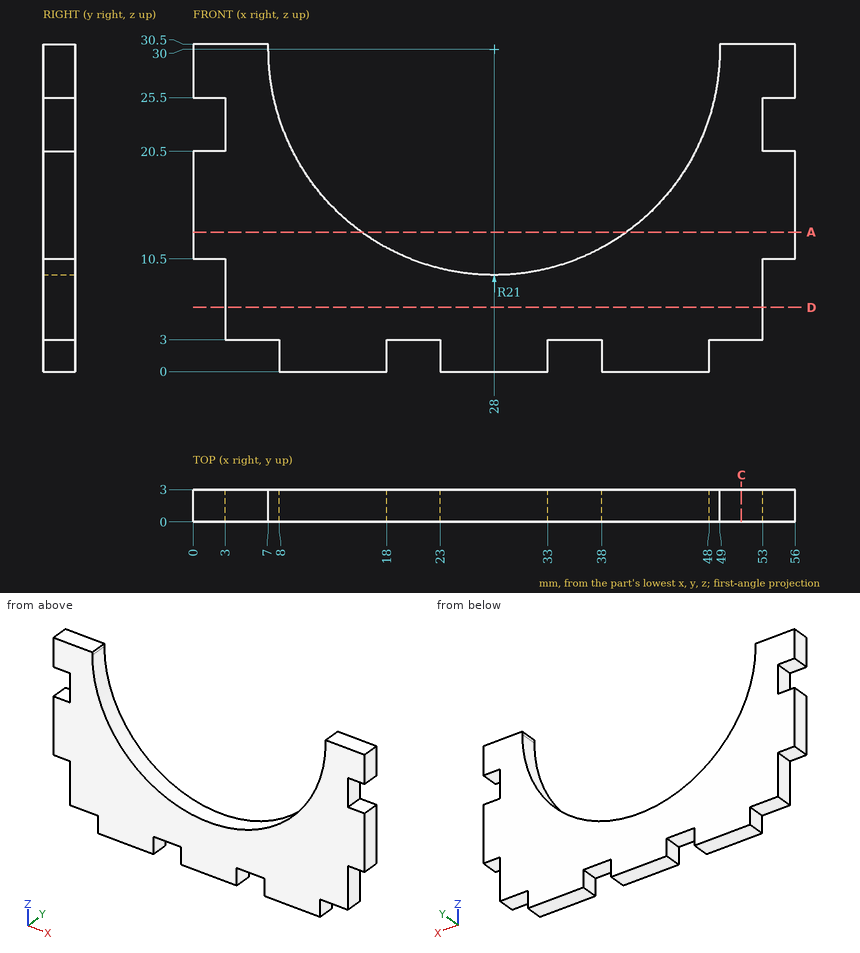
Print and shaded views of the part. All mm, measured from the part's lowest x, y and z. Round coordinates to 2 decimals unless told otherwise and drop trailing zeros. Write each loop counter-clockwise with the first axis right and the second up, starting at its lowest first coordinate (ties: lowest second). Pieces come first, ordered by that corner, then holes. Notation, with made-up numbers: (-1, 10) - (4, 10) arc R21 cw to (4, 27) - close; hole circle Ø7 at (30.25, -37.5). An arc over 180 degrees is marked (long way). Write each question's results on one line, items separated by ' | '. Start each with the question number.
Item 1: Wall check: L1, parallel to X at y = 2, z = 2.5; L2, parallel to X at y = 2.45, z = 12.5; L3, parallel to X at y = 0.1, z = 19. Give the ranges that are in metal, low to high. Write a range as [from, to].
Item 2: Saw through at D-D (z = 6). Write the cut outline in (x, y).
Item 3: Saw through at A-A (z = 13). Write the cut outline in (x, y), and give its area (3 significant figures).
Item 4: Drop flat-ended pins along their axis: P1, Ø1.5, axis at y = 2, z = 2, coming from the -X side; P2, Ø0.9, axis at y = 2, z = 5, coming from the +X side; P3, Ø1.5, axis at x = 20.5, y = 2, coming from the -Z side; P4, Ø12, axis at x = 38, z = 25, coming from the +Y side. Give the stop position or say it passes through.
Item 5: Saw through at C-C (x = 51). Write the cut outline in (y, z).
Results are:
1) L1: x = [8, 18], [23, 33], [38, 48] | L2: x = [0, 16.39], [39.61, 56] | L3: x = [0, 10.11], [45.89, 56]
2) outline: (3, 0) - (53, 0) - (53, 3) - (3, 3) - close
3) outline: (0, 0) - (15.67, 0) - (15.67, 3) - (0, 3) - close; (40.33, 0) - (56, 0) - (56, 3) - (40.33, 3) - close | area: 94.0 mm²
4) P1: stops at x = 8 | P2: stops at x = 53 | P3: stops at z = 3 | P4: passes through
5) outline: (0, 3) - (3, 3) - (3, 30.5) - (0, 30.5) - close
